Could you check a few things on this model? Use its own coordinates, in mm. Round coordinates to 2 decimals unless told otherwise and drop trailing zeros. Loops run counter-clockwise (first coordinate to the right, second up) from the corner with the lowest first, then second, coordinate; pieces in that order, holes last. Notation, with made-up numbers: (87, 42) - (139, 42) arc R21 ccw to (139, 56) - close; hole circle Ø5 at (28, 0.5). An arc over 180 degrees is marked (long way). Put each result on its own line as item: value. Start each with the question number.
from build123d import *

# Parameters (mm, degrees)
ESBO_O1_W                = 78
ESBO_O1_H                = 20
RESSALTO_EXTRUS_O1_DEPTH = 8
ESBO_O2_W                = 2.8
ESBO_O2_H                = 2.8
CORTE_EXTRUS_O1_DEPTH    = 45.55333882


with BuildPart() as part:
    # Esboço1 → Ressalto-extrusão1 (new body)
    with BuildSketch(Plane.XY):
        Rectangle(ESBO_O1_W, ESBO_O1_H)
        with BuildLine():
            Line((-31, 7), (31, 7))
            ThreePointArc((31, 7), (34.535533906, 5.535533906), (36, 2))
            Line((36, 2), (36, -2))
            ThreePointArc((36, -2), (34.535533906, -5.535533906), (31, -7))
            Line((31, -7), (-31, -7))
            ThreePointArc((-31, -7), (-34.535533906, -5.535533906), (-36, -2))
            Line((-36, -2), (-36, 2))
            ThreePointArc((-36, 2), (-34.535533906, 5.535533906), (-31, 7))
        make_face(mode=Mode.SUBTRACT)
    extrude(amount=RESSALTO_EXTRUS_O1_DEPTH)

    # Esboço2 → Corte-extrusão1 (cut, through all)
    with BuildSketch(Plane(origin=(0, 10, 0), x_dir=(1, 0, 0), z_dir=(0, 1, 0))):
        with Locations((-8, -4)):
            Rectangle(ESBO_O2_W, ESBO_O2_H)
        with Locations((0, -4)):
            Rectangle(ESBO_O2_W, ESBO_O2_H)
        with Locations((-16, -4)):
            Rectangle(ESBO_O2_W, ESBO_O2_H)
        with Locations((-24, -4)):
            Rectangle(ESBO_O2_W, ESBO_O2_H)
        with Locations((24, -4)):
            Rectangle(ESBO_O2_W, ESBO_O2_H)
        with Locations((16, -4)):
            Rectangle(ESBO_O2_W, ESBO_O2_H)
        with Locations((8, -4)):
            Rectangle(ESBO_O2_W, ESBO_O2_H)
    extrude(amount=-CORTE_EXTRUS_O1_DEPTH, mode=Mode.SUBTRACT)


solid = part.part
Item 1: Suppose I cut it at D-D, the plane y = 7.75. Count the separate pieces of the cut face and the enclosed holes in it, then the cut area to 3 significant figures.
Item 2: I need wall thicknesses on line 1 (Y direction, x = -26, z = 4.5); line 2 (X direction, y = 0.5, z = 1.25); line 3 (X direction, y = -4.5, z = 5.75). Which ranges of each line are inside material? Lowest first, please. Write a range as from..to.
Item 3: Suppose I cut it at B-B, the plane z = 6.25. List the corners of the cut face in (x, y) for me, then the cut area to 3 significant figures.
Item 4: Suppose I cut it at A-A, the plane y = -1.25. List the corners of the cut face in (x, z) for me.
Item 5: Suppose I cut it at C-C, the plane x = 13. List the corners of the cut face in (y, z) for me, then the cut area to 3 significant figures.
Numbers:
1. separate pieces: 1
1. enclosed holes: 7
1. area: 569 mm^2
2. line 1: -10..-7, 7..10
2. line 2: -39..-36, 36..39
2. line 3: -39..-35.33, 35.33..39
3. outline: (-39, -10) - (39, -10) - (39, 10) - (-39, 10) - close; hole (-36, -2) arc R5 ccw to (-31, -7) - (31, -7) arc R5 ccw to (36, -2) - (36, 2) arc R5 ccw to (31, 7) - (-31, 7) arc R5 ccw to (-36, 2) - close
3. area: 573 mm^2
4. outline: (-39, 0) - (-36, 0) - (-36, 8) - (-39, 8) - close; (36, 0) - (39, 0) - (39, 8) - (36, 8) - close
5. outline: (-10, 0) - (-7, 0) - (-7, 8) - (-10, 8) - close; (7, 0) - (10, 0) - (10, 8) - (7, 8) - close
5. area: 48.0 mm^2
